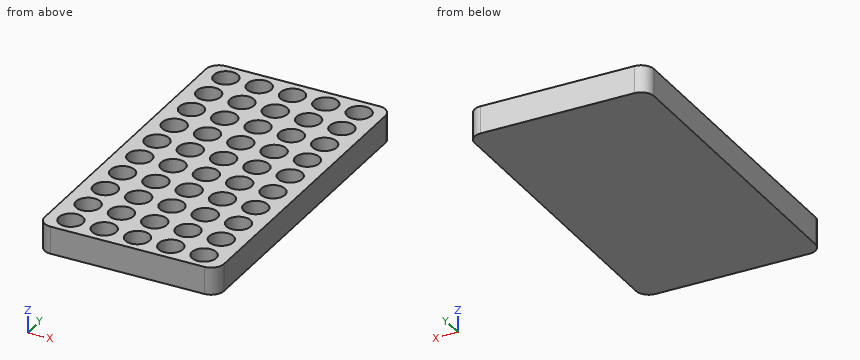
```python
from build123d import *

# Parameters (mm, degrees)
F0_R     = 6
F1_DEPTH = 12.7
F3_DEPTH = 0.9


with BuildPart() as f1:
    # F0 (on Top) → F1 (new body)
    with BuildSketch(Plane.XY):
        with BuildLine():
            Line((38.1, 81.28), (-38.1, 81.28))
            ThreePointArc((-38.1, 81.28), (-42.590128, 79.420128), (-44.45, 74.93))
            Line((-44.45, 74.93), (-44.45, -74.93))
            ThreePointArc((-44.45, -74.93), (-42.590128, -79.420128), (-38.1, -81.28))
            Line((-38.1, -81.28), (38.1, -81.28))
            ThreePointArc((38.1, -81.28), (42.590128, -79.420128), (44.45, -74.93))
            Line((44.45, -74.93), (44.45, 74.93))
            ThreePointArc((44.45, 74.93), (42.590128, 79.420128), (38.1, 81.28))
        make_face()
        with Locations((-33.02, -72)):
            Circle(F0_R, mode=Mode.SUBTRACT)
        with Locations((-33.02, -56)):
            Circle(F0_R, mode=Mode.SUBTRACT)
        with Locations((-16.51, -72)):
            Circle(F0_R, mode=Mode.SUBTRACT)
        with Locations((-16.51, -56)):
            Circle(F0_R, mode=Mode.SUBTRACT)
        with Locations((-33.02, -40)):
            Circle(F0_R, mode=Mode.SUBTRACT)
        with Locations((-33.02, -24)):
            Circle(F0_R, mode=Mode.SUBTRACT)
        with Locations((-33.02, -8)):
            Circle(F0_R, mode=Mode.SUBTRACT)
        with Locations((-16.51, -40)):
            Circle(F0_R, mode=Mode.SUBTRACT)
        with Locations((-16.51, -24)):
            Circle(F0_R, mode=Mode.SUBTRACT)
        with Locations((-16.51, -8)):
            Circle(F0_R, mode=Mode.SUBTRACT)
        with Locations((0, -72)):
            Circle(F0_R, mode=Mode.SUBTRACT)
        with Locations((16.51, -72)):
            Circle(F0_R, mode=Mode.SUBTRACT)
        with Locations((0, -56)):
            Circle(F0_R, mode=Mode.SUBTRACT)
        with Locations((16.51, -56)):
            Circle(F0_R, mode=Mode.SUBTRACT)
        with Locations((33.02, -72)):
            Circle(F0_R, mode=Mode.SUBTRACT)
        with Locations((33.02, -56)):
            Circle(F0_R, mode=Mode.SUBTRACT)
        with Locations((0, -40)):
            Circle(F0_R, mode=Mode.SUBTRACT)
        with Locations((0, -24)):
            Circle(F0_R, mode=Mode.SUBTRACT)
        with Locations((16.51, -40)):
            Circle(F0_R, mode=Mode.SUBTRACT)
        with Locations((16.51, -24)):
            Circle(F0_R, mode=Mode.SUBTRACT)
        with Locations((0, -8)):
            Circle(F0_R, mode=Mode.SUBTRACT)
        with Locations((16.51, -8)):
            Circle(F0_R, mode=Mode.SUBTRACT)
        with Locations((33.02, -40)):
            Circle(F0_R, mode=Mode.SUBTRACT)
        with Locations((33.02, -24)):
            Circle(F0_R, mode=Mode.SUBTRACT)
        with Locations((33.02, -8)):
            Circle(F0_R, mode=Mode.SUBTRACT)
        with Locations((-33.02, 8)):
            Circle(F0_R, mode=Mode.SUBTRACT)
        with Locations((-33.02, 24)):
            Circle(F0_R, mode=Mode.SUBTRACT)
        with Locations((-33.02, 40)):
            Circle(F0_R, mode=Mode.SUBTRACT)
        with Locations((-16.51, 8)):
            Circle(F0_R, mode=Mode.SUBTRACT)
        with Locations((-16.51, 24)):
            Circle(F0_R, mode=Mode.SUBTRACT)
        with Locations((-16.51, 40)):
            Circle(F0_R, mode=Mode.SUBTRACT)
        with Locations((-33.02, 56)):
            Circle(F0_R, mode=Mode.SUBTRACT)
        with Locations((-33.02, 72)):
            Circle(F0_R, mode=Mode.SUBTRACT)
        with Locations((-16.51, 56)):
            Circle(F0_R, mode=Mode.SUBTRACT)
        with Locations((-16.51, 72)):
            Circle(F0_R, mode=Mode.SUBTRACT)
        with Locations((0, 8)):
            Circle(F0_R, mode=Mode.SUBTRACT)
        with Locations((16.51, 8)):
            Circle(F0_R, mode=Mode.SUBTRACT)
        with Locations((0, 24)):
            Circle(F0_R, mode=Mode.SUBTRACT)
        with Locations((0, 40)):
            Circle(F0_R, mode=Mode.SUBTRACT)
        with Locations((16.51, 24)):
            Circle(F0_R, mode=Mode.SUBTRACT)
        with Locations((16.51, 40)):
            Circle(F0_R, mode=Mode.SUBTRACT)
        with Locations((33.02, 8)):
            Circle(F0_R, mode=Mode.SUBTRACT)
        with Locations((33.02, 24)):
            Circle(F0_R, mode=Mode.SUBTRACT)
        with Locations((33.02, 40)):
            Circle(F0_R, mode=Mode.SUBTRACT)
        with Locations((0, 56)):
            Circle(F0_R, mode=Mode.SUBTRACT)
        with Locations((16.51, 56)):
            Circle(F0_R, mode=Mode.SUBTRACT)
        with Locations((0, 72)):
            Circle(F0_R, mode=Mode.SUBTRACT)
        with Locations((16.51, 72)):
            Circle(F0_R, mode=Mode.SUBTRACT)
        with Locations((33.02, 56)):
            Circle(F0_R, mode=Mode.SUBTRACT)
        with Locations((33.02, 72)):
            Circle(F0_R, mode=Mode.SUBTRACT)
    extrude(amount=F1_DEPTH)

    # F2 (on face) → F3 (join)
    with BuildSketch(Plane(origin=(0, 0, 0), x_dir=(1, 0, 0), z_dir=(0, 0, -1))):
        with BuildLine():
            Line((38.1, 81.28), (-38.1, 81.28))
            ThreePointArc((-38.1, 81.28), (-42.590128, 79.420128), (-44.45, 74.93))
            Line((-44.45, 74.93), (-44.45, -74.93))
            ThreePointArc((-44.45, -74.93), (-42.590128, -79.420128), (-38.1, -81.28))
            Line((-38.1, -81.28), (38.1, -81.28))
            ThreePointArc((38.1, -81.28), (42.590128, -79.420128), (44.45, -74.93))
            Line((44.45, -74.93), (44.45, 74.93))
            ThreePointArc((44.45, 74.93), (42.590128, 79.420128), (38.1, 81.28))
        make_face()
    extrude(amount=F3_DEPTH)


solid = f1.part
```
Read the model definition and answer for the solid it produces. Units are mm, in the model's axes. Give positions to 0.01 mm unless a question says otherwise; leave off trailing zeros. Write each loop counter-clockwise with the first axis right and the second up, starting at its lowest first coordinate (ties: lowest second). Pieces come first, ordered by that corner, then holes. Notation, with made-up numbers: (-19.75, 40.5) - (-14.75, 40.5) arc R19 cw to (-14.75, 56.5) - close; hole circle Ø7 at (-18.75, 36). An arc over 180 degrees is marked (long way). Write item = value, one per line. Start each with the question number.
Item 1: Find the intervals of material crossed by probe 1 along X at (y, z) = (-25, 4); probe 2 along X at (y, z) = (-21, 10.5); probe 3 along Z at (x, y) = (-33, 73.5), in increasing order. Write a range as [from, to].
Item 2: This flat-tipped pin is pushed along its axis until it touches: P1, Ø3.5, axis at x = -35.5, y = -24.5, coming from the +Z side. Where does it stop, or does it pass through?
Item 3: Find section B-B (z = 7.25). State how many separate pieces and enclosed holes the cut face has, then the cut area to 3 significant figures.
Item 4: Find section C-C (y = -43). Give the vertices of the cut face in (x, z), then the cut area to 3 significant figures.
Item 5: Find section A-A (y = 56). Give the vertices of the cut face in (x, z), then the cut area to 3 significant figures.
Response:
q1.probe_1 = [-44.45, -38.94], [-27.1, -22.43], [-10.59, -5.92], [5.92, 10.59], [22.43, 27.1], [38.94, 44.45]
q1.probe_2 = [-44.45, -38.22], [-27.82, -21.71], [-11.31, -5.2], [5.2, 11.31], [21.71, 27.82], [38.22, 44.45]
q1.probe_3 = [-0.9, 0]
q2.P1 = 0
q3.separate_pieces = 1
q3.enclosed_holes = 50
q3.area = 8,760 mm²
q4.outline = (-44.45, -0.9) - (44.45, -0.9) - (44.45, 12.7) - (38.22, 12.7) - (38.22, 0) - (27.82, 0) - (27.82, 12.7) - (21.71, 12.7) - (21.71, 0) - (11.31, 0) - (11.31, 12.7) - (5.2, 12.7) - (5.2, 0) - (-5.2, 0) - (-5.2, 12.7) - (-11.31, 12.7) - (-11.31, 0) - (-21.71, 0) - (-21.71, 12.7) - (-27.82, 12.7) - (-27.82, 0) - (-38.22, 0) - (-38.22, 12.7) - (-44.45, 12.7) - close
q4.area = 549 mm²
q5.outline = (-44.45, -0.9) - (44.45, -0.9) - (44.45, 12.7) - (39.02, 12.7) - (39.02, 0) - (27.02, 0) - (27.02, 12.7) - (22.51, 12.7) - (22.51, 0) - (10.51, 0) - (10.51, 12.7) - (6, 12.7) - (6, 0) - (-6, 0) - (-6, 12.7) - (-10.51, 12.7) - (-10.51, 0) - (-22.51, 0) - (-22.51, 12.7) - (-27.02, 12.7) - (-27.02, 0) - (-39.02, 0) - (-39.02, 12.7) - (-44.45, 12.7) - close
q5.area = 447 mm²
